```python
from build123d import *

# Parameters (mm, degrees)
SKETCH2_W           = 23
SKETCH2_H           = 10
BOSS_EXTRUDE1_DEPTH = 40
SKETCH3_R           = 2.5
CUT_EXTRUDE1_DEPTH  = 43.804789452
SKETCH4_W           = 150
SKETCH4_H           = 5
BOSS_EXTRUDE2_DEPTH = 70
SKETCH5_W           = 23
SKETCH5_H           = 10
BOSS_EXTRUDE3_DEPTH = 5


with BuildPart() as part:
    # Sketch2 → Boss-Extrude1 (new body)
    with BuildSketch(Plane(origin=(0, 0, 0), x_dir=(1, 0, 0), z_dir=(0, 1, 0))):
        Rectangle(SKETCH2_W, SKETCH2_H)
    extrude(amount=BOSS_EXTRUDE1_DEPTH)

    # Sketch3 → Cut-Extrude1 (cut, through all)
    with BuildSketch(Plane.XY.offset(5)):
        with Locations((0, 32)):
            Circle(SKETCH3_R)
        with Locations((0, 22)):
            Circle(SKETCH3_R)
    extrude(amount=-CUT_EXTRUDE1_DEPTH, mode=Mode.SUBTRACT)



with BuildPart() as body_2:
    # Sketch4 → Boss-Extrude2 (new body)
    with BuildSketch(Plane.XY.offset(5)):
        with Locations((-63.5, -2.5)):
            Rectangle(SKETCH4_W, SKETCH4_H)
    extrude(amount=BOSS_EXTRUDE2_DEPTH)


with BuildPart() as part_1:
    add(part.part)

    add(body_2.part)  # Boss-Extrude3 merges body 2
    # Sketch5 → Boss-Extrude3 (add)
    with BuildSketch(Plane.XZ):
        Rectangle(SKETCH5_W, SKETCH5_H)
    extrude(amount=BOSS_EXTRUDE3_DEPTH)


solid = part_1.part
```
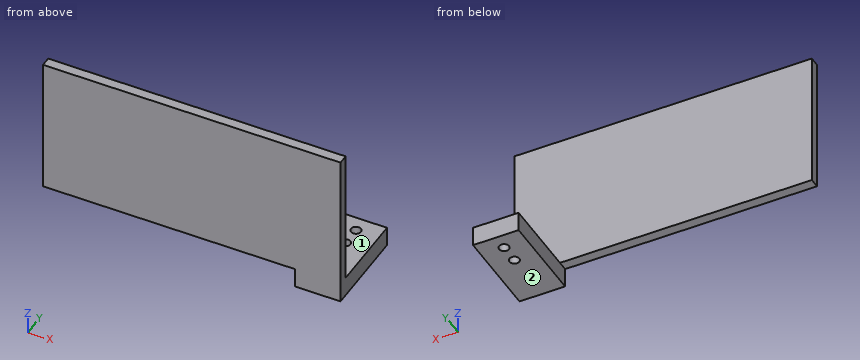
Design review of the part built by this model. Coordinates are the model's own, in mm. Face numbers are marked on the shaded views. A direction names the side the tool comes from. Round coordinates to 2 decimals unless told otherwise and drop trailing zeros. Write each loop counter-clockwise with the first axis right and the second up, starting at its lowest first coordinate (ties: lowest second). Pieces come first, ordered by that corner, then holes.
Item 1: We need section C-C on z = 32. Write out the cut boundary in (x, y), and give its area (3 significant figures).
Item 2: For the marked faces 1 and 2, list the 3-axis set-ups (+Z, -Z, +X, -X, +Y, -Y) from which the entire face can be reached by the end or side of a thin tool; tool diameter is ignored.
Item 3: We need section D-D on y = -2. Write out the cut boundary in (x, z).
Item 4: We need section A-A on y = 22. Write out the cut boundary in (x, z).
Item 5: Clearance check with flat-ended pins moving along their axes: pin 1 Ø8 at (y, z) = (12, 1.5) entering from -X; pin 2 Ø1.5 at (x, y) = (-72.5, -2.5) entering from -Z; pin 3 Ø11.5 at (x, y) = (-4, 23) entering from +Z. State where each tip first meets the part, or that it passes through.
Item 6: For probe 1 along Y at (x, z) = (0, 1.75); probe 2 along Z at (x, y) = (-71, -3); probe 3 along Y at (x, z) = (-14.5, 42), list the stretches that pass through material, from the lowest coordinate up.
Item 7: We need section B-B on x = 0. Write out the cut boundary in (y, z).
Returned:
1. outline: (-138.5, -5) - (11.5, -5) - (11.5, 0) - (-138.5, 0) - close
1. area: 750 mm2
2. face 1: +Z, +X, -X, +Y
2. face 2: -Z, +X, -X, +Y, -Y
3. outline: (-138.5, 5) - (-11.5, 5) - (-11.5, -5) - (11.5, -5) - (11.5, 75) - (-138.5, 75) - close
4. outline: (-11.5, -5) - (-2.5, -5) - (-2.5, 5) - (-11.5, 5) - close; (2.5, -5) - (11.5, -5) - (11.5, 5) - (2.5, 5) - close
5. pin 1: stops at x = -11.5
5. pin 2: stops at z = 5
5. pin 3: stops at z = 5
6. probe 1: y = -5 to 19.5, 24.5 to 29.5, 34.5 to 40
6. probe 2: z = 5 to 75
6. probe 3: y = -5 to 0
7. outline: (-5, -5) - (19.5, -5) - (19.5, 5) - (0, 5) - (0, 75) - (-5, 75) - close; (24.5, -5) - (29.5, -5) - (29.5, 5) - (24.5, 5) - close; (34.5, -5) - (40, -5) - (40, 5) - (34.5, 5) - close
